Verification items for the finished model (mm, model axes). Coordinates: 2 decimals unless noted, no trailing zeros. Answer as a JSON object with one key per item and string values. Group by question number.
Q1. Cross-section at A-A on z = 40.5. Give the number of separate pieces and of enclosed holes in the cut face, and give its area (3 significant figures).
Q2. Gauge pin test, flat ends, axial feed: pin 1 Ø2 at (y, z) = (0.5, -39) entering from -X; pin 2 Ø1.5 at (x, z) = (-1.5, -1) entering from +Y; pin 3 Ø4.5 at (y, z) = (0, 39) entering from +X. Record the tip position at first contact, or that the pin passes through.
Q3. Scan lines: L1, parallel to Y at x = 0, z = 1; L2, parallel to Y at x = 1.75, z = 110; L3, parallel to X at y = 10.75, z = -19. Record each from-to range of solid material in increasing order.
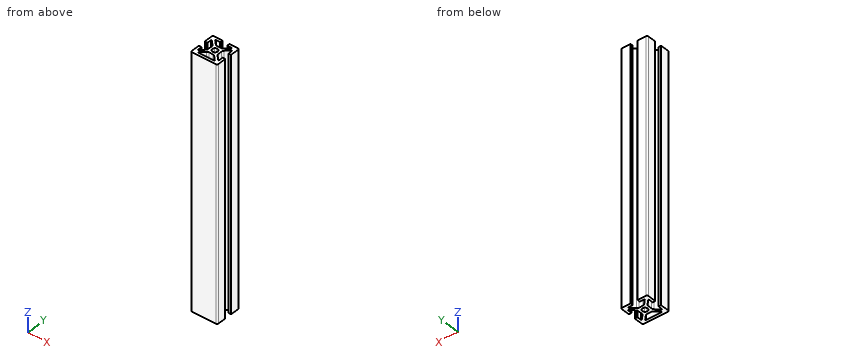
```python
from build123d import *

# Parameters (mm, degrees)
BOSS_EXTRUDE1_DEPTH = 120.65
FILLET2_R           = 0.254
FILLET1_R           = 1.27
SKETCH5_W           = 7.112
SKETCH5_H           = 2.54
BOSS_EXTRUDE2_DEPTH = 241.3


with BuildPart() as part:
    # Sketch3 → Boss-Extrude1 (new body, symmetric)
    with BuildSketch(Plane.XY):
        with BuildLine():
            Line((-12.7, 12.7), (-1.796051224, 1.796051224))
            ThreePointArc((-1.796051224, 1.796051224), (-0.972015918, 2.346654013), (0, 2.54))
            Line((0, 2.54), (0, 4.826))
            Line((0, 4.826), (-1.977846327, 4.826))
            ThreePointArc((-1.977846327, 4.826), (-2.949862246, 5.019345987), (-3.773897552, 5.569948776))
            Line((-3.773897552, 5.569948776), (-7.772528286, 9.56857951))
            ThreePointArc((-7.772528286, 9.56857951), (-7.847628361, 9.946133082), (-7.527553898, 10.16))
            Line((-7.527553898, 10.16), (-3.302, 10.16))
            Line((-3.302, 10.16), (-3.302, 12.7))
            Line((-3.302, 12.7), (-12.7, 12.7))
        make_face()
    extrude(amount=BOSS_EXTRUDE1_DEPTH, both=True)

    # Fillet2
    fillet2_edges = [part.edges().sort_by_distance(p)[0] for p in [
        (-3.302, 12.7, 0),
        (-3.302, 10.16, 0),
    ]]
    fillet(fillet2_edges, radius=FILLET2_R)

    # Mirror1: part across plane


with BuildPart() as part_1:
    add(part.part)
    add(part.part.mirror(Plane(origin=(0, 0, 120.65), x_dir=(0, 0, 1), z_dir=(0.707106781, 0.707106781, 0))))

    # Fillet1
    fillet1_edges = [part_1.edges().sort_by_distance(p)[0] for p in [
        (-12.7, 12.7, 0),
    ]]
    fillet(fillet1_edges, radius=FILLET1_R)

    # Mirror2: part across plane


with BuildPart() as part_2:
    add(part_1.part)
    add(part_1.part.mirror(Plane(origin=(0, 0, 120.65), x_dir=(0, 0, 1), z_dir=(0, 1, 0))))

    # Mirror5: part across plane


with BuildPart() as part_3:
    add(part_2.part)
    add(part_2.part.mirror(Plane(origin=(0, 0, 120.65), x_dir=(0, 0, 1), z_dir=(-1, 0, 0))))

    # Sketch5 → Boss-Extrude2 (add, through all)
    with BuildSketch(Plane.XY.offset(120.65)):
        with Locations((0, -11.43)):
            Rectangle(SKETCH5_W, SKETCH5_H)
    extrude(amount=-BOSS_EXTRUDE2_DEPTH)


solid = part_3.part
```
Computed values:
{
 "1": {"separate pieces": "1", "enclosed holes": "2", "area": "332 mm²"},
 "2": {"pin 1": "stops at x = -4.83", "pin 2": "stops at y = 4.84", "pin 3": "stops at x = 4.84"},
 "3": {"L1": "y = -12.7 to -10.16, -4.83 to -2.54, 2.54 to 4.83", "L2": "y = -12.7 to -10.16, -4.83 to -1.84, 1.84 to 4.83", "L3": "x = -12.7 to -3.3, 3.3 to 12.7"}
}
